Verification items for this drawing (mm, ordinates from the low corner). A direction names the side the tool comes from. Give positions to 0.01 mm unless a question says otherwise; leave off trailing zeros. Loops run counter-clockwise (first coordinate to the right, second up) from the corner with the lowest first, then second, coordinate; pieces in that order, holes last. Notation, with made-up numbers: (39, -35.75) -> (69, -35.75) arc R19 cw to (69, 0.25) -> close; hole circle Ø6 at (76.5, 58). An arc over 180 degrees is marked (long way). Answer as CSV lines item,"result". Start each with the question number.
(1) Section check A-A on x = 5. Enter the section's corners in (y, z).
(2) Material ranges on line 1 (Y direction, x = 9.25, z = 5.5); line 2 (X direction, y = 99, z = 6); line 3 (Z direction, x = 7, y = 91.5), recorded low to high. Write a range as from..to.
(3) Section check C-C on y = 86. Enter the section's corners in (x, z), plus the area to 3 significant figures.
(4) Access from +Z, -Z, +X, -X, +Y, -Y to the whole of each face (thin tool, end or side, straight path). Record for the marked faces 1 and 2.
(5) Gauge pin test, flat ends, axial feed: pin 1 Ø3 at (y, z) = (89.5, 4) entering from -X; pin 2 Ø1 at (y, z) = (54.5, 3) entering from -X; pin 3 Ø6 at (y, z) = (17, 3.5) entering from +X; pin 4 Ø2 at (x, z) = (8.5, 1) entering from +Y. Record the tip position at first contact, or that the pin passes through.
(6) Section check B-B on z = 5. Enter the section's corners in (x, y), plus the area to 3 significant figures.
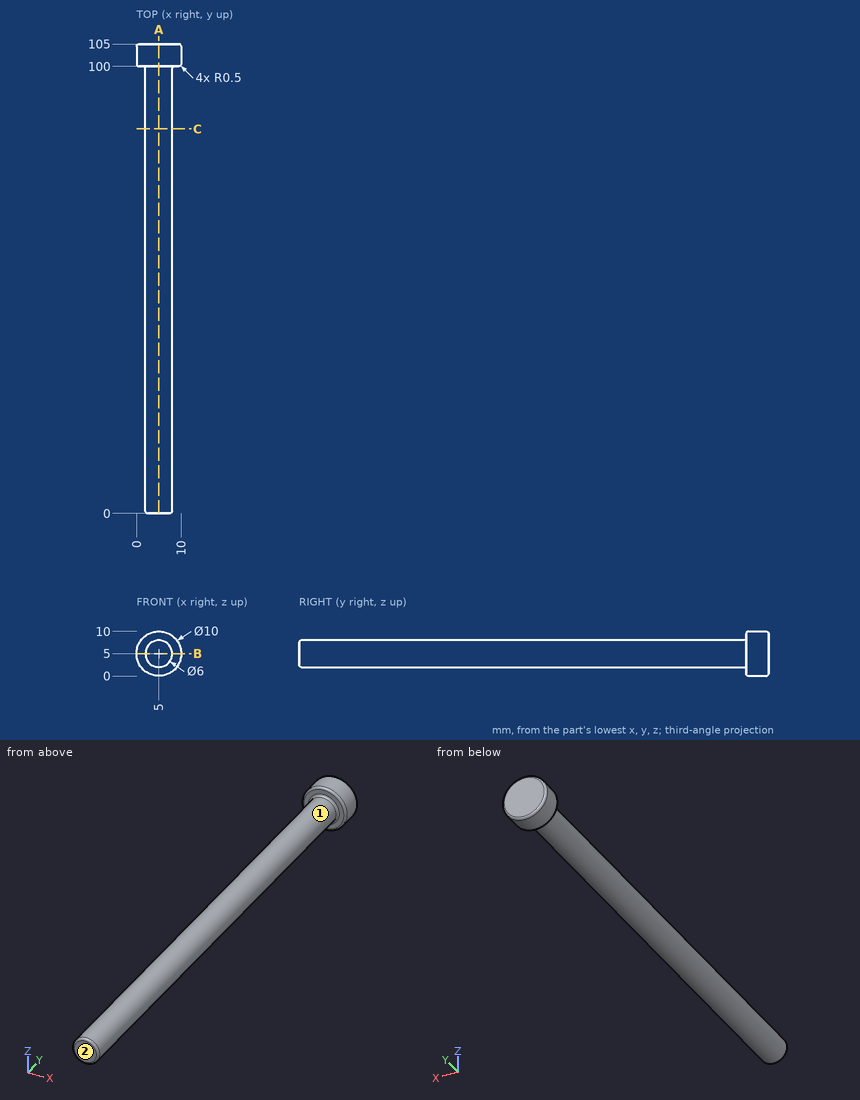
Working result:
1,outline,"(0, 2.5) arc R0.5 ccw to (0.5, 2) -> (99.5, 2) arc R0.5 cw to (100, 1.5) -> (100, 0.5) arc R0.5 ccw to (100.5, 0) -> (104.5, 0) arc R0.5 ccw to (105, 0.5) -> (105, 9.5) arc R0.5 ccw to (104.5, 10) -> (100.5, 10) arc R0.5 ccw to (100, 9.5) -> (100, 8.5) arc R0.5 cw to (99.5, 8) -> (0.5, 8) arc R0.5 ccw to (0, 7.5) -> close"
2,line 1,"y = 100..105"
2,line 2,"x = 2.17..7.83"
2,line 3,"z = 2.76..7.24"
3,outline,"circle Ø6 at (5, 5)"
3,area,"28.3 mm^2"
4,face 1,"-Y"
4,face 2,"+Z, -Z, +X, -X, -Y"
5,pin 1,"stops at x = 2"
5,pin 2,"stops at x = 2.4"
5,pin 3,"stops at x = 8"
5,pin 4,"stops at y = 105"
6,outline,"(0, 100.5) arc R0.5 ccw to (0.5, 100) -> (1.5, 100) arc R0.5 cw to (2, 99.5) -> (2, 0.5) arc R0.5 ccw to (2.5, 0) -> (7.5, 0) arc R0.5 ccw to (8, 0.5) -> (8, 99.5) arc R0.5 cw to (8.5, 100) -> (9.5, 100) arc R0.5 ccw to (10, 100.5) -> (10, 104.5) arc R0.5 ccw to (9.5, 105) -> (0.5, 105) arc R0.5 ccw to (0, 104.5) -> close"
6,area,"650 mm^2"
